```python
from build123d import *

# Parameters (mm, degrees)
SKETCH_1_W             = 22
SKETCH_1_H             = 134.5
EXTRUDE_1_DEPTH        = 8
HOLE_WIZARD_M5_1_D     = 4.2
HOLE_WIZARD_M5_1_DEPTH = 12.4
HOLE_WIZARD_M5_1_TIP   = 1.2618073
SKETCH_6_W             = 22
SKETCH_6_H             = 8
EXTRUDE_2_DEPTH        = 12
SKETCH_7_R             = 2.75
CUT_EXTRUDE_1_DEPTH    = 9


with BuildPart() as part:
    # 草图1 → 凸台-拉伸1 (new body)
    with BuildSketch(Plane.XY):
        with Locations((11, 67.25)):
            Rectangle(SKETCH_1_W, SKETCH_1_H)
    extrude(amount=EXTRUDE_1_DEPTH)

    # M5 螺纹孔1
    with Locations(Plane(origin=(0, 134.5, 0), x_dir=(1, 0, 0), z_dir=(0, 1, 0))):
        with Locations((17, -4), (5, -4)):
            Hole(HOLE_WIZARD_M5_1_D / 2, depth=HOLE_WIZARD_M5_1_DEPTH)
            with Locations((0, 0, -(HOLE_WIZARD_M5_1_DEPTH + HOLE_WIZARD_M5_1_TIP / 2))):  # 118° drill point
                Cone(0, HOLE_WIZARD_M5_1_D / 2, HOLE_WIZARD_M5_1_TIP, mode=Mode.SUBTRACT)

    # 草图6 → 凸台-拉伸2 (add)
    with BuildSketch(Plane.XY.offset(8)):
        with Locations((11, 4)):
            Rectangle(SKETCH_6_W, SKETCH_6_H)
    extrude(amount=EXTRUDE_2_DEPTH)

    # 草图7 → 切除-拉伸1 (cut, through all)
    with BuildSketch(Plane(origin=(0, 8, 0), x_dir=(1, 0, 0), z_dir=(0, 1, 0))):
        with Locations((5, -14)):
            Circle(SKETCH_7_R)
        with Locations((17, -14)):
            Circle(SKETCH_7_R)
    extrude(amount=-CUT_EXTRUDE_1_DEPTH, mode=Mode.SUBTRACT)


solid = part.part
```
Check sheet for the modelled part. Datum: model origin and axes. Units: mm. A direction names the side the tool comes from. Round coordinates to 2 decimals unless told otherwise and drop trailing zeros. Order: outer loops, then holes, each group sorted by start corner. A loop starts at its lowest first (then second) coordinate and runs counter-clockwise, first axis right, second up. Notation, with made-up numbers: (80.5, 43) - (139.5, 43) arc R10 cw to (139.5, 48) - close; hole circle Ø11 at (15.25, 69.25). An arc over 180 degrees is marked (long way). Write item = value, one per line.
Q1. Section check B-B (y = 115.5). Record the boundary of the cut face in (x, z).
Computed:
outline = (0, 0) - (22, 0) - (22, 8) - (0, 8) - close
Q2. Go/stop test with flat-tipped pins: pin 1 (12 mm diameter, centred on y = 88, z = 4.5, fed in from -X); pin 2 (3.5 mm diameter, centred on x = 13.5, z = 12.5, fed in from +Y); pin 3 (2.5 mm diameter, centred on x = 17, z = 4, fed in from +Y); pin 4 (5 mm diameter, centred on x = 5, z = 14, fed in from -Y). Record where each tip stops, or that it passes through.
Computed:
pin_1 = 0
pin_2 = 8
pin_3 = 121.59
pin_4 = through
Q3. Tool access check on faces 4 (the face through (15.06, 128.21, 4.8)), 5 (the face through (22, 66, 5)). Record the directions out of +Z, -Z, +X, -X, +Y, -Y that give a thin tool (end or side, any length) a straight path to the whole face; none if there is none.
Computed:
face_4 = +Y
face_5 = +Z, -Z, +X, +Y, -Y
Q4. Section check A-A (z = 14). Record the boundary of the cut face in (x, y), and give its area (3 significant figures).
Computed:
outline = (0, 0) - (2.25, 0) - (2.25, 8) - (0, 8) - close; (7.75, 0) - (14.25, 0) - (14.25, 8) - (7.75, 8) - close; (19.75, 0) - (22, 0) - (22, 8) - (19.75, 8) - close
area = 88.0 mm^2
Q5. Draft check along Z on faces 1 (the face through (11, 72, 8)), 2 (the face through (16.636, 121.057, 3.984)), 3 (the face through (11, 8, 14)). Enter one of: pulls with the +Z half, pulls with the -Z half, needs draft (parallel to the pull), parting line crosses it, or undercut.
Computed:
face_1 = pulls with the +Z half
face_2 = undercut
face_3 = needs draft
Q6. Thickness scan on line 1 along X through (y, z) = (4, 14); line 2 along Z through (x, y) = (5, 4.5); line 3 along Z through (x, y) = (9.25, 128.5). Record the ranges inside material, lowest first.
Computed:
line_1 = 0 to 2.25, 7.75 to 14.25, 19.75 to 22
line_2 = 0 to 11.25, 16.75 to 20
line_3 = 0 to 8
